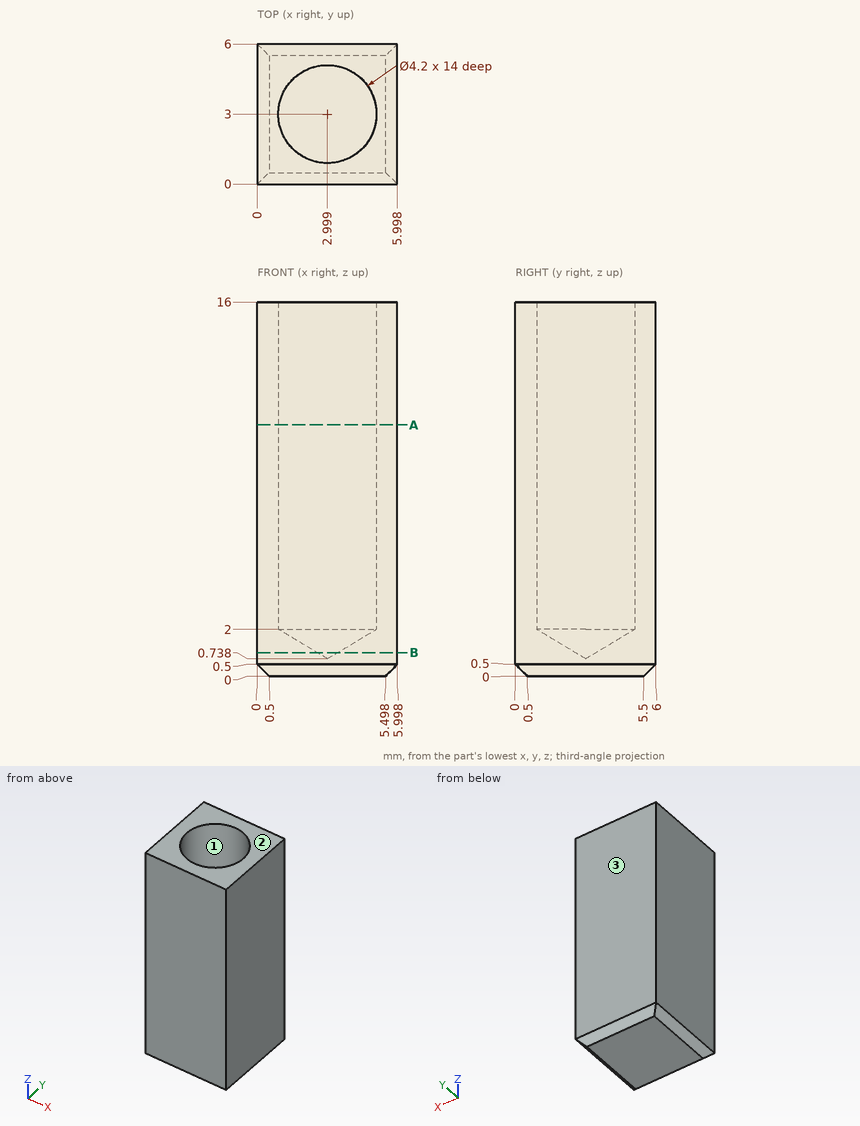
Geometry check sheet. Reference: drawing and pictorial views, mm from the part's lowest x, y, z. Round coordinates to 2 decimals unless told otherwise and drop trailing zeros. Write each loop counter-clockwise with the first axis right and the second up, starting at its lowest first coordinate (ties: lowest second). Pieces come first, ordered by that corner, then holes. Notation, with made-up numbers: (66, -26) -> (122, -26) arc R15 ccw to (122, -2) -> close; hole circle Ø9 at (-22.75, -14.5). An arc over 180 degrees is marked (long way). Answer as CSV lines item,"result". Start each with the question number.
1) Material ranges on line 1 (X direction, y = 3, z = 4.5); line 2 (Y direction, x = 1.5, z = 7.25), recorded low to high. Write a range as from..to.
2) Go/stop test with a flat-tipped pin: P1, Ø3.5, axis at x = 3, y = 3, coming from the +Z side. Record where the tip stops, or that it passes through.
3) Section check A-A on z = 10.75. Enter the section's corners in (x, y), and give its area (3 significant figures).
4) Release check for a two-part mould opening along Y. For the marked faces 1, 2 and 3 record: pulls with the +Y half, pulls with the -Y half, needs draft (parallel to the pull), parting line crosses it, or undercut.
5) Section check B-B on z = 1. Enter the section's corners in (x, y) (1 decimal), and give its area (3 significant figures).
Found:
1,line 1,"x = 0..0.9, 5.1..6"
1,line 2,"y = 0..1.53, 4.47..6"
2,P1,"stops at z = 1.79"
3,outline,"(0, 0) -> (6, 0) -> (6, 6) -> (0, 6) -> close; hole circle Ø4.2 at (3, 3)"
3,area,"22.1 mm^2"
4,face 1,"undercut"
4,face 2,"needs draft"
4,face 3,"pulls with the +Y half"
5,outline,"(0, 0) -> (6, 0) -> (6, 6) -> (0, 6) -> close; hole circle Ø0.9 at (3, 3)"
5,area,"35.4 mm^2"
